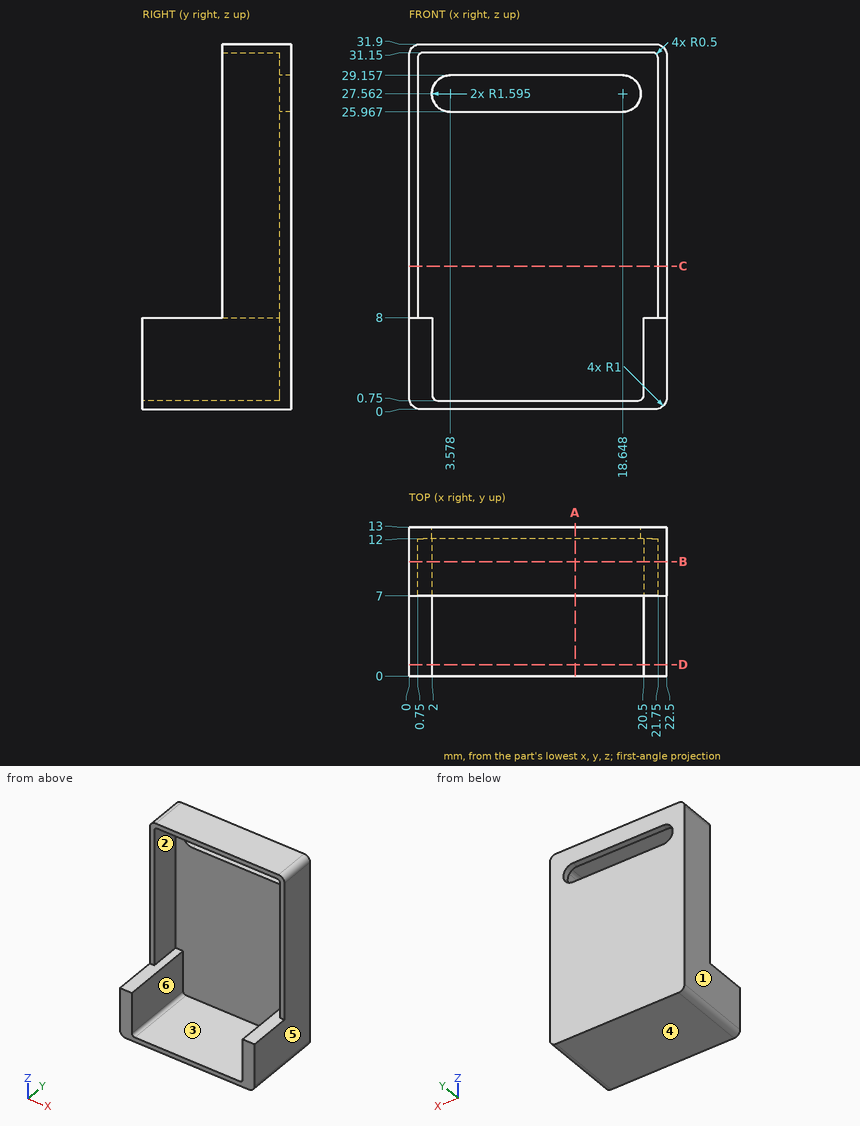
For this review, use the dimensioned drawing (mm, ordinates from the lowest corner) and the shaded views. A direction names the side the tool comes from. Give positions to 0.01 mm unless a question says otherwise; leave off trailing zeros. Order: outer loops, then holes, each group sorted by start corner. A loop starts at its lowest first (then second) coordinate and runs counter-clockwise, first axis right, second up. Notation, with made-up numbers: (51, -25) - (79, -25) arc R8 cw to (79, -15) - close; hole circle Ø11 at (72, 58). An arc over 180 degrees is marked (long way). Use a Markdown table: item, result. Add a question column.
(1) Machinability: for the marked faces 1 and 2, which of the approach directions +Z, -Z, +X, -X, +Y, -Y give a long, thin tool a straight path to every point of the face, cutting with its end or side? Answer none if there is none.
(2) Wall thickness on probe 1 along Z at (x, y) = (3, 8.5); probe 2 along X at (y, z) = (11.5, 3); probe 3 along X at (y, z) = (8.75, 14): over which ranges is each line inside the solid? List them lowest first. Write a range as [from, to].
(3) Mouldability with a two-part tool opening along X and no side actions: class the marked faces 3, 4, 5 and 6 as +X half, -X half, draft (parallel to the pull), parting line (faces both ways), or undercut.
(4) Add section C-C on z = 12.5. Give the boundary of the cut face in (x, y), then the cut area to 3 significant figures.
(5) Add section D-D on y = 1. Give the boundary of the cut face in (x, z).
(6) Clearance check with flat-ended pins moving along their axes: P1, Ø1.6, axis at x = 1, y = 5.5, coming from the +Z side; P2, Ø6.5, axis at x = 9.5, z = 21.5, coming from the -Y side. State where each tip first meets the part, or that it passes through.
(7) Add section A-A on x = 14.5. Give the boundary of the cut face in (y, z).
(8) Add section B-B on y = 10. Give the boundary of the cut face in (x, z).
Report:
| question | item | result |
|---|---|---|
| 1 | face 1 | +Z, -Z, -X, +Y, -Y |
| 1 | face 2 | -Y |
| 2 | probe 1 | z = [0, 0.75], [31.15, 31.9] |
| 2 | probe 2 | x = [0, 2], [20.5, 22.5] |
| 2 | probe 3 | x = [0, 0.75], [21.75, 22.5] |
| 3 | face 3 | undercut |
| 3 | face 4 | draft |
| 3 | face 5 | +X half |
| 3 | face 6 | undercut |
| 4 | outline | (0, 7) - (0.75, 7) - (0.75, 12) - (21.75, 12) - (21.75, 7) - (22.5, 7) - (22.5, 13) - (0, 13) - close |
| 4 | area | 30.0 mm² |
| 5 | outline | (0, 1) arc R1 ccw to (1, 0) - (21.5, 0) arc R1 ccw to (22.5, 1) - (22.5, 8) - (20.5, 8) - (20.5, 1.25) arc R0.5 cw to (20, 0.75) - (2.5, 0.75) arc R0.5 cw to (2, 1.25) - (2, 8) - (0, 8) - close |
| 6 | P1 | stops at z = 8 |
| 6 | P2 | stops at y = 12 |
| 7 | outline | (0, 0) - (13, 0) - (13, 25.97) - (12, 25.97) - (12, 0.75) - (0, 0.75) - close; (7, 31.15) - (12, 31.15) - (12, 29.16) - (13, 29.16) - (13, 31.9) - (7, 31.9) - close |
| 8 | outline | (0, 1) arc R1 ccw to (1, 0) - (21.5, 0) arc R1 ccw to (22.5, 1) - (22.5, 30.9) arc R1 ccw to (21.5, 31.9) - (1, 31.9) arc R1 ccw to (0, 30.9) - close; hole (0.75, 8) - (2, 8) - (2, 1.25) arc R0.5 ccw to (2.5, 0.75) - (20, 0.75) arc R0.5 ccw to (20.5, 1.25) - (20.5, 8) - (21.75, 8) - (21.75, 30.65) arc R0.5 ccw to (21.25, 31.15) - (1.25, 31.15) arc R0.5 ccw to (0.75, 30.65) - close |
